Verification items for this drawing (mm, ordinates from the low corner). A direction names the side the tool comes from. Round coordinates to 2 decimals unless told otherwise and drop trailing zeros. Order: outer loops, then holes, each group sorted by start corner. A loop starts at its lowest first (then second) coordinate and runs counter-clockwise, first axis right, second up. Notation, with made-up numbers: (53, -24.5) -> (57, -24.5) arc R18 ccw to (57, -11.5) -> close; hole circle Ø3 at (-15, -24). An arc over 180 degrees is marked (long way). Return JSON: item names as keys, results as strings. Group by question number.
Item 1: Access from +Z, -Z, +X, -X, +Y, -Y to the whole of each face (thin tool, end or side, straight path). Record for the marked faces 5 and 6.
Item 2: Sectioned sample at C-C on y = 1.5. Record the cut outline in (x, z), plus the area to 3 significant figures.
Item 3: Depth check by flat-ended pin: pin 1 Ø1 at (x, z) = (13, 8) entering from +Y; pin 2 Ø1.5 at (x, y) = (17, 4.5) entering from -Z; pin 3 Ø3 at (x, y) = (17.5, 5.5) entering from +Z. Enter the tip coordinate at first touch or a pass-through.
Item 4: Scan lines: probe 1 along X at (y, z) = (2.35, 10); probe 2 along X at (y, z) = (5.7, 10); probe 3 along Z at (x, y) = (6.25, 2.75). Record each from-to range of solid material in increasing order. Write a range as from..to.
Item 5: Draft check along Z on the marked faces 1, 2, 3 and 4. Enter one of: pulls with the +Z half, pulls with the -Z half, needs draft (parallel to the pull), parting line crosses it, or undercut.
Item 6: Sectioned sample at A-A on z = 10. Record the cut outline in (x, y).
Item 7: Sectioned sample at B-B on x = 13.25. Record the cut outline in (y, z).
Item 8: Sectioned sample at D-D on x = 17.25. Record the cut outline in (y, z), plus the area to 3 significant figures.
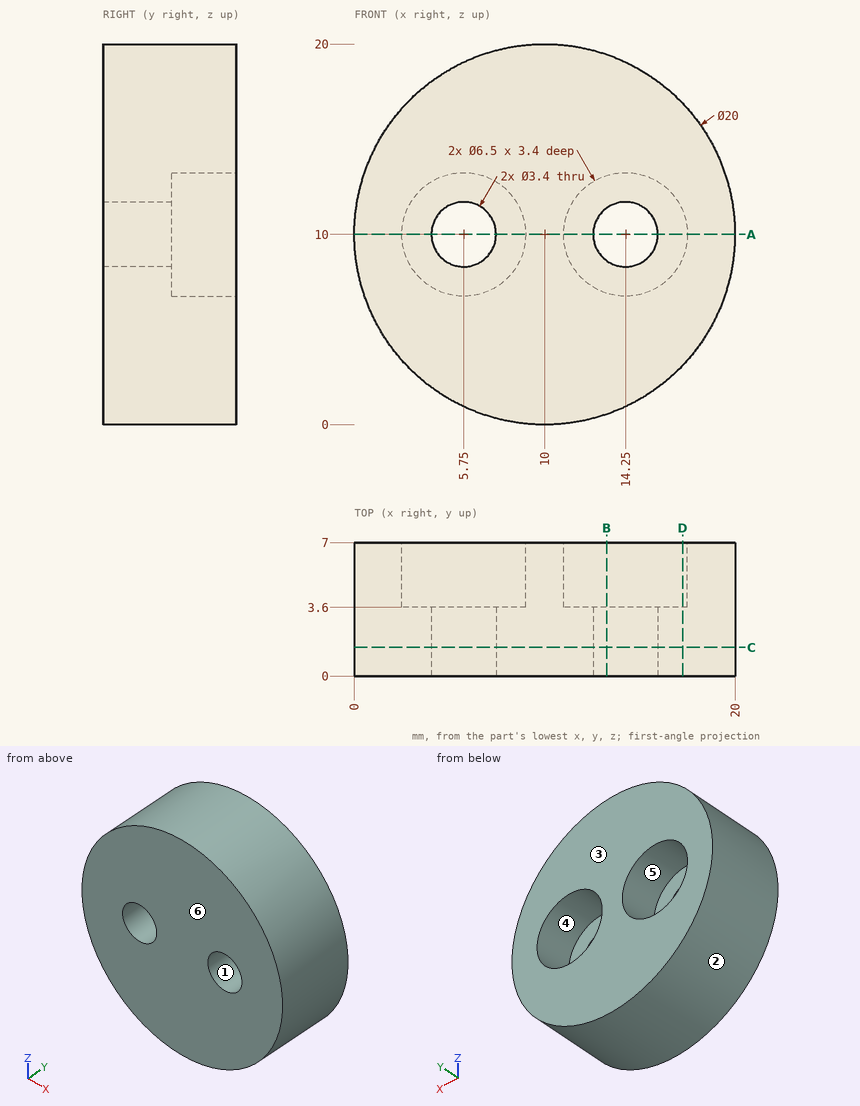
Recorded:
{
 "1": {"face 5": "+Y", "face 6": "+Z, -Z, +X, -X, -Y"},
 "2": {"outline": "circle Ø20 at (10, 10); hole circle Ø3.4 at (5.75, 10); hole circle Ø3.4 at (14.25, 10)", "area": "296 mm²"},
 "3": {"pin 1": "y = 3.6", "pin 2": "z = 2.19", "pin 3": "z = 18"},
 "4": {"probe 1": "0..4.05, 7.45..12.55, 15.95..20", "probe 2": "0..2.5, 9..11, 17.5..20", "probe 3": "0.73..8.38, 11.62..19.27"},
 "5": {"face 1": "undercut", "face 2": "parting line crosses it", "face 3": "needs draft", "face 4": "undercut"},
 "6": {"outline": "(0, 0) -> (4.05, 0) -> (4.05, 3.6) -> (2.5, 3.6) -> (2.5, 7) -> (0, 7) -> close; (7.45, 0) -> (12.55, 0) -> (12.55, 3.6) -> (11, 3.6) -> (11, 7) -> (9, 7) -> (9, 3.6) -> (7.45, 3.6) -> close; (15.95, 0) -> (20, 0) -> (20, 7) -> (17.5, 7) -> (17.5, 3.6) -> (15.95, 3.6) -> close"},
 "7": {"outline": "(0, 0.54) -> (7, 0.54) -> (7, 6.91) -> (3.6, 6.91) -> (3.6, 8.63) -> (0, 8.63) -> close; (0, 11.37) -> (3.6, 11.37) -> (3.6, 13.09) -> (7, 13.09) -> (7, 19.46) -> (0, 19.46) -> close"},
 "8": {"outline": "(0, 3.11) -> (7, 3.11) -> (7, 8.75) -> (3.6, 8.75) -> (3.6, 11.25) -> (7, 11.25) -> (7, 16.89) -> (0, 16.89) -> close", "area": "87.9 mm²"}
}
